The model under review builds one solid part; all positions refer to its coordinate system, in mm. Face numbers are marked on the shaded views. A direction names the side the tool comes from. Round coordinates to 2 decimals unless told otherwise and drop trailing zeros. Loops run counter-clockwise (first coordinate to the right, second up) from the corner with the lowest first, then second, coordinate; pieces in that order, holes last. Notation, with made-up numbers: M 3.25,35 L 45.25,35 A31 ccw 45.25,74 Z; hole C 43,81 d1. An arc over 180 degrees is marked long. One line per question, with ' | ' between items.
from build123d import *

# Parameters (mm, degrees)
EXTRUDE_1_DEPTH     = 10
SKETCH_2_R          = 2.5
SKETCH_2_R_2        = 2
CUT_EXTRUDE_1_DEPTH = 40


with BuildPart() as part:
    # 草图1 → 凸台-拉伸1 (new body)
    with BuildSketch(Plane(origin=(0, 0, 0), x_dir=(1, 0, 0), z_dir=(0, 1, 0))):
        with BuildLine():
            Line((-25, 0), (-34, 0))
            Line((-34, 0), (-34, 30))
            Line((-34, 30), (-26, 30))
            ThreePointArc((-26, 30), (-20.276357576, 26.094481357), (-13.388178788, 26.846911717))
            ThreePointArc((-13.388178788, 26.846911717), (-8.812963312, 28.676326084), (-4, 29.732137495))
            Line((-4, 29.732137495), (4, 29.732137495))
            ThreePointArc((4, 29.732137495), (8.812963312, 28.676326084), (13.388178788, 26.846911717))
            ThreePointArc((13.388178788, 26.846911717), (20.276357576, 26.094481357), (26, 30))
            Line((26, 30), (34, 30))
            Line((34, 30), (34, 0))
            Line((34, 0), (25, 0))
            ThreePointArc((25, 0), (0, 25), (-25, 0))
        make_face()
    extrude(amount=EXTRUDE_1_DEPTH)

    # 草图2 → 切除-拉伸1 (cut)
    with BuildSketch(Plane(origin=(0, 0, -30), x_dir=(-1, 0, 0), z_dir=(0, 0, -1))):
        with Locations((-29.5, 5)):
            Circle(SKETCH_2_R)
        with Locations((29.5, 5)):
            Circle(SKETCH_2_R)
        with Locations((0, 5)):
            Circle(SKETCH_2_R_2)
    extrude(amount=-CUT_EXTRUDE_1_DEPTH, mode=Mode.SUBTRACT)


solid = part.part
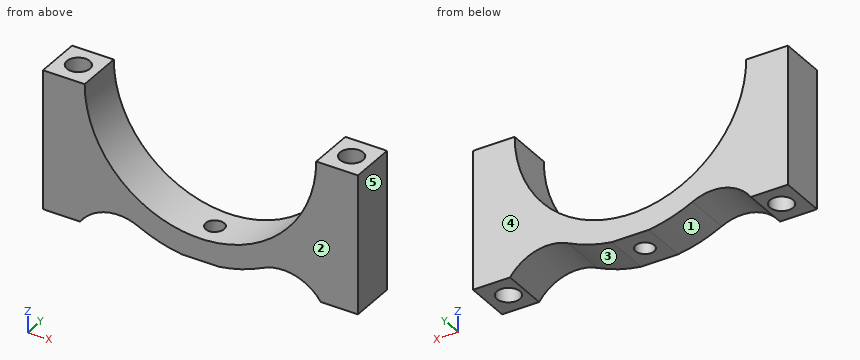
1) Machinability: for the marked faces 1 and 2, which of the approach directions +Z, -Z, +X, -X, +Y, -Y give a long, thin tool a straight path to every point of the face, cutting with its end or side? Answer none if there is none.
Output values:
face 1: -Z, +Y, -Y | face 2: +Z, -Z, +X, -X, -Y
2) Mouldability with a two-part tool opening along X and no side actions: class the marked faces 3, 4 and 5 as +X half, -X half, draft (parallel to the pull), parting line (faces both ways), or undercut.
Output values:
face 3: undercut | face 4: draft | face 5: +X half
3) Add section A-A on y = 5. State the section outline as (x, z) points, then the cut area to 3 significant figures.
Output values:
outline: M -34,-30 L -32,-30 L -32,0 L -34,0 Z; M -27,-30 L -26,-30 A10 cw -13.39,-26.85 A30 ccw -4,-29.73 L -2,-29.73 L -2,-24.92 A25 cw -25,0 L -27,0 Z; M 2,-29.73 L 4,-29.73 A30 ccw 13.39,-26.85 A10 cw 26,-30 L 27,-30 L 27,0 L 25,0 A25 cw 2,-24.92 Z; M 32,-30 L 34,-30 L 34,0 L 32,0 Z | area: 628 mm²
4) Add section D-D on y = 9. State the section outline as (x, z) points.
Output values:
outline: M -34,-30 L -26,-30 A10 cw -13.39,-26.85 A30 ccw -4,-29.73 L 4,-29.73 A30 ccw 13.39,-26.85 A10 cw 26,-30 L 34,-30 L 34,0 L 25,0 A25 cw -25,0 L -34,0 Z
5) For line 1 (X direction, y = 5.25, z = -25.5); line 2 (Y direction, x = 0, z = -26); line 3 (Y direction, x = -29.5, z = -23.5), list the stretches that pass through material, from the lowest coordinate up.
Output values:
line 1: x = -34 to -31.99, -27.01 to -1.98, 1.98 to 27.01, 31.99 to 34 | line 2: y = 0 to 3, 7 to 10 | line 3: y = 0 to 2.5, 7.5 to 10
6) Add section B-B on z = -5. State the section outline as (x, y) points.
Output values:
outline: M -34,0 L -24.49,0 L -24.49,10 L -34,10 Z; M 24.49,0 L 34,0 L 34,10 L 24.49,10 Z; hole C -29.5,5 d5; hole C 29.5,5 d5
7) Add section C-C on x = -29.5. State the section outline as (y, z) points, then the cut area to 3 significant figures.
Output values:
outline: M 0,-30 L 2.5,-30 L 2.5,0 L 0,0 Z; M 7.5,-30 L 10,-30 L 10,0 L 7.5,0 Z | area: 150 mm²
8) Insertion check: P1, Ø1.5, axis at x = 9, y = 4.5, coming from the -Z side; P2, Ø1.5, axis at x = 0, y = 6.5, coming from the +Z side; P3, Ø2.5, axis at x = 0.5, y = 4, coming from the -Z side. Each pin has a flat end and moves straight along its axis. Give the tip position at first contact, or say it passes through.
Output values:
P1: stops at z = -28.84 | P2: stops at z = -24.99 | P3: stops at z = -29.73
